The drawing under review shows one solid part. Ordinate dimensions are in mm from its lowest x, y, z. Round coordinates to 2 decimals unless told otherwise and drop trailing zeros. Order: outer loops, then holes, each group sorted by start corner. A loop starts at its lowest first (then second) coordinate and runs counter-clockwise, first axis right, second up.
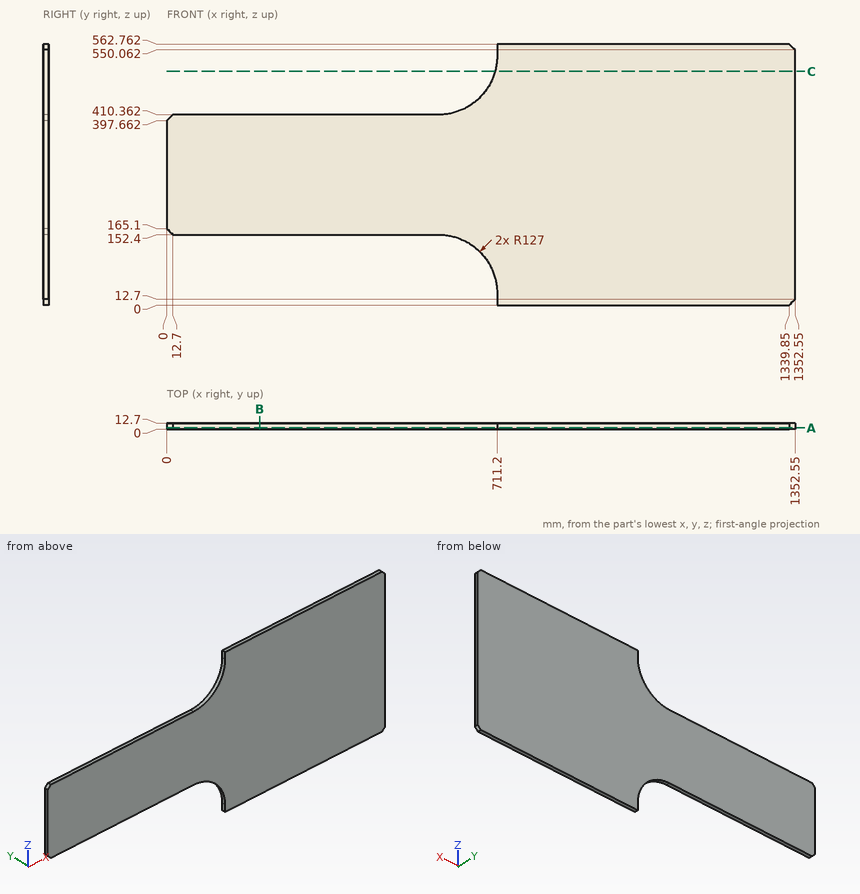
(1) To check wall thickness, follow L1, parallel to Z at x = 431, y = 4.75; L2, parallel to Z at x = 627.5, y = 0.5; L3, parallel to X at y = 7, z = 27. State the ranges of each line that lie inside material, in increasing order.
(2) We need section A-A (y = 3). Give the boundary of the cut face in (x, z), and give its area (3 significant figures).
(3) We need section B-B (x = 199.5). Give the boundary of the cut face in (y, z), and give its area (3 significant figures).
(4) We need section C-C (z = 504). Give the boundary of the cut face in (x, y), and give its area (3 significant figures).
(5) Clearance check with flat-ended pins moving along their axes: P1, Ø3, axis at y = 6, z = 436.5, coming from the -X side; P2, Ø4, axis at x = 361, y = 3.5, coming from the +Z side; P3, Ø2, axis at y = 10.5, z = 92.5, coming from the -X side; P4, Ø1, axis at y = 3.5, z = 312, coming from the -X side. State where each tip first meets the part, or that it passes through.
Verdict:
1. L1: z = 152.4 to 410.36
1. L2: z = 144.79 to 417.97
1. L3: x = 711.19 to 1352.55
2. outline: (0, 165.1) - (12.7, 152.4) - (584.2, 152.4) arc R127 cw to (711.2, 25.4) - (711.2, 0) - (1339.85, 0) - (1352.55, 12.7) - (1352.55, 550.06) - (1339.85, 562.76) - (711.2, 562.76) - (711.2, 537.36) arc R127 cw to (584.2, 410.36) - (12.7, 410.36) - (0, 397.66) - close
2. area: 551,000 mm2
3. outline: (0, 152.4) - (12.7, 152.4) - (12.7, 410.36) - (0, 410.36) - close
3. area: 3,280 mm2
4. outline: (706.74, 0) - (1352.55, 0) - (1352.55, 12.7) - (706.74, 12.7) - close
4. area: 8,200 mm2
5. P1: stops at x = 659.37
5. P2: stops at z = 410.36
5. P3: stops at x = 691.4
5. P4: stops at x = 0
